Build history of the part. All positions in model axes, mm. A direction names the side the tool comes from. Round coordinates to 2 decimals unless told otherwise and drop trailing zeros. Write each loop counter-clockwise with the first axis right and the second up, starting at its lowest first coordinate (ties: lowest second). Pieces come first, ordered by that corner, then holes. Notation, with made-up numbers: M 30.5,-40 L 71.5,-40 A32 cw 71.5,-8 Z; hole C 17,-6.5 d3. An arc over 180 degrees is marked long. Write item = value, one per line.
from build123d import *

# Parameters (mm, degrees)
F0_W     = 24
F0_H     = 6
F0_H_2   = 10
F1_DEPTH = 17.4
F2_R     = 8
F3_R     = 2
F5_R     = 5.5
F6_DEPTH = 25
F7_R     = 1
F4_W     = 17.4
F4_H     = 8.7
F8_DEPTH = 18
F9_R     = 8.69999


# Not quite as in the source:
# - a fillet or chamfer is up to 0.001 mm smaller than in the source, because OpenCascade refuses the exact size


with BuildPart() as f1:
    # F0 (on Top) → F1 (new body)
    with BuildSketch(Plane.XY):
        Polygon((3, 41.0029157541), (3, 47.0029157541), (-3, 47.0029157541), (-3, -48.9970842459), (3, -48.9970842459), (3, -38.9970842459), align=None)
        with Locations((15, 44.0029157541)):
            Rectangle(F0_W, F0_H)
        with Locations((15, -43.9970842459)):
            Rectangle(F0_W, F0_H_2)
    extrude(amount=F1_DEPTH)

    # F2
    f2_edges = [f1.edges().sort_by_distance(p)[0] for p in [
        (-3, 47.002916, 8.7),
        (-3, -48.997084, 8.7),
    ]]
    fillet(f2_edges, radius=F2_R)

    # F3
    f3_edges = [f1.edges().sort_by_distance(p)[0] for p in [
        (3, 41.002916, 8.7),
    ]]
    fillet(f3_edges, radius=F3_R)

    # F5 (on face) → F6 (cut)
    with BuildSketch(Plane.XZ.offset(48.9970842459)):
        with Locations((17, 8.7)):
            Circle(F5_R)
    extrude(amount=-F6_DEPTH, mode=Mode.SUBTRACT)

    # F7
    f7_edges = [f1.edges().sort_by_distance(p)[0] for p in [
        (3, -38.997084, 8.7),
    ]]
    fillet(f7_edges, radius=F7_R)

    # F4 (on face) → F8 (join)
    with BuildSketch(Plane(origin=(0, 47.0029157541, 0), x_dir=(-1, 0, 0), z_dir=(0, 1, 0))):
        with Locations((-18.3, 13.05)):
            Rectangle(F4_W, F4_H)
    extrude(amount=F8_DEPTH)

    # F9 (radius 8.7 in the source; OpenCascade refuses exactly that, so slightly less here)
    f9_edges = [f1.edges().sort_by_distance(p)[0] for p in [
        (27, 65.002916, 13.05),
        (9.6, 65.002916, 13.05),
    ]]
    fillet(f9_edges, radius=F9_R)


solid = f1.part
1. Band-saw the part on B-B (x = 17). List the corners of the cut face in (y, z).
Responses:
outline = M -49,0 L -39,0 L -39,3.2 L -49,3.2 Z; M -49,14.2 L -39,14.2 L -39,17.4 L -49,17.4 Z; M 41,0 L 47,0 L 47,8.7 L 64.91,8.7 L 64.91,17.4 L 41,17.4 Z
2. Tool access for faces 1 (the face through (9.6, 52, 13)), 2 (the face through (16, 41.003, 9)), 3 (the face through (16.284, -44.067, 14.153)): list every direction of +Z, -Z, +X, -X, +Y, -Y with a clear straight run to the whole face (end or side of a thin tool).
Responses:
face_1 = +Z, -Z, -X, +Y
face_2 = +Z, -Z, +X
face_3 = -Y
3. Flat gauge pins, fed straight in: pin 1 (4.5 mm diameter, centred on y = 50.5, z = 14.5, fed in from -X); pin 2 (5 mm diameter, centred on x = 22, y = 53, fed in from -Z); pin 3 (1 mm diameter, centred on x = 20, z = 5.5, fed in from +Y). Where does each tip first touch, or does it go through?
Responses:
pin_1 = 9.6
pin_2 = 8.7
pin_3 = 47
4. Mould opens along Y. For faces 4 (the face through (3, 0, 9)), 5 (the face through (-0.719, 44.597, 8.822)), 6 (the face through (12.8, -38.997, 4.7)), 7 (the face through (2, 0, 0)) say: pulls with the +Y half, pulls with the -Y half, needs draft (parallel to the pull), parting line crosses it, or undercut.
Responses:
face_4 = undercut
face_5 = pulls with the +Y half
face_6 = undercut
face_7 = needs draft
5. Band-saw the part on D-D (x = 23.75). List the corners of the cut face in (y, z), plus the area to 3 significant figures.
Responses:
outline = M -49,0 L -39,0 L -39,17.4 L -49,17.4 Z; M 41,0 L 47,0 L 47,8.7 L 63.08,8.7 L 63.08,17.4 L 41,17.4 Z
area = 418 mm²
6. Probe probe 1 along Z at (x, y) = (17, -41); probe 2 along Y at (x, z) = (23, 1); probe 3 along X at (y, z) = (-22.5, 6.5). List the from-to ranges inside material, lowest first.
Responses:
probe_1 = 0 to 3.2, 14.2 to 17.4
probe_2 = -49 to -39, 41 to 47
probe_3 = -3 to 3
